Check sheet for the modelled part. Datum: model origin and axes. Units: mm. Face numbers are marked on the shaded views. A direction names the side the tool comes from. Round coordinates to 2 decimals unless told otherwise and drop trailing zeros. Order: outer loops, then holes, each group sorted by start corner. A loop starts at its lowest first (then second) coordinate and runs counter-clockwise, first axis right, second up. Notation, with made-up numbers: M -25,-18.75 L -17,-18.75 A12 ccw -17,-3.75 Z; hole C 61.5,79.25 d3. An arc over 180 degrees is marked long. One line per item, written item: value. Start each with the question number.
(1) Thickness scan on L1, parallel to X at y = 0, z = 14.5; L2, parallel to X at y = 3, z = 11; L3, parallel to X at y = -0.75, z = 30. Record the ranges inside material, lowest first.
(2) Depth check by flat-ended pin: pin 1 Ø7 at (x, y) = (20, 0) entering from -Z; pin 2 Ø3 at (x, y) = (-1.5, -0.5) entering from -Z. Enter the tip coordinate at first touch or a pass-through.
(3) Cross-section at B-B, the plane y = 0. Enter the section's corners in (x, z), and give its area (3 significant figures).
(4) Cross-section at D-D, the plane y = 4. Enter the section's corners in (x, z).
(5) Cross-section at A-A, the plane z = 14.5. Enter the section's corners in (x, y).
(6) Release check for a two-part mould opening along Y. For the marked faces 3, 4 and 5 record: released by +Y, released by -Y, zero draft, split by the parting line, or undercut.
(7) Access from +Z, -Z, +X, -X, +Y, -Y to the whole of each face (thin tool, end or side, straight path). Record for the marked faces 1 and 2.
(8) Cross-section at C-C, the plane x = 21. Enter the section's corners in (y, z).
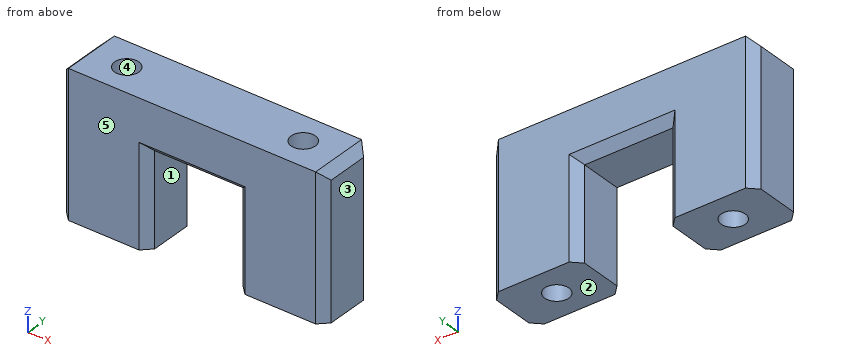
from build123d import *

# Parameters (mm, degrees)
SKETCH1_W           = 13.5
SKETCH1_H           = 60
SKETCH1_R           = 2.75
BOSS_EXTRUDE1_DEPTH = 32.5
SKETCH2_W           = 20
SKETCH2_H           = 21
CUT_EXTRUDE1_DEPTH  = 14.5
CHAMFER1_SIZE       = 2
CHAMFER2_SIZE       = 2


with BuildPart() as part:
    # Sketch1 → Boss-Extrude1 (new body)
    with BuildSketch(Plane(origin=(0, 0, 0), x_dir=(0, 1, 0), z_dir=(0, 0, 1))):
        Rectangle(SKETCH1_W, SKETCH1_H)
        with Locations((0, 20)):
            Circle(SKETCH1_R, mode=Mode.SUBTRACT)
        with Locations((0, -20)):
            Circle(SKETCH1_R, mode=Mode.SUBTRACT)
    extrude(amount=BOSS_EXTRUDE1_DEPTH)

    # Sketch2 → Cut-Extrude1 (cut, through all)
    with BuildSketch(Plane(origin=(0, 6.75, 0), x_dir=(-1, 0, 0), z_dir=(0, 1, 0))):
        with Locations((0, 10.5)):
            Rectangle(SKETCH2_W, SKETCH2_H)
    extrude(amount=-CUT_EXTRUDE1_DEPTH, mode=Mode.SUBTRACT)

    # Chamfer1
    chamfer1_edges = [part.edges().sort_by_distance(p)[0] for p in [
        (30, 0, 32.5),
        (30, 6.75, 16.25),
        (30, -6.75, 16.25),
        (-30, -6.75, 16.25),
        (-30, 6.75, 16.25),
        (-30, 0, 32.5),
    ]]
    chamfer(chamfer1_edges, length=CHAMFER1_SIZE)

    # Chamfer2
    chamfer2_edges = [part.edges().sort_by_distance(p)[0] for p in [
        (10, -6.75, 10.5),
        (0, -6.75, 21),
        (-10, -6.75, 10.5),
        (10, 6.75, 10.5),
        (-10, 6.75, 10.5),
        (0, 6.75, 21),
    ]]
    chamfer(chamfer2_edges, length=CHAMFER2_SIZE)


solid = part.part
Values found:
1. L1: -30 to -22.75, -17.25 to -10, 10 to 17.25, 22.75 to 30
1. L2: -30 to -10, 10 to 30
1. L3: -30 to -22.65, -17.35 to 17.35, 22.65 to 30
2. pin 1: z = 0
2. pin 2: z = 21
3. outline: M -30,0 L -22.75,0 L -22.75,32.5 L -28,32.5 L -30,30.5 Z; M -17.25,0 L -10,0 L -10,21 L 10,21 L 10,0 L 17.25,0 L 17.25,32.5 L -17.25,32.5 Z; M 22.75,0 L 30,0 L 30,30.5 L 28,32.5 L 22.75,32.5 Z
3. area: 1,170 mm^2
4. outline: M -30,0 L -10,0 L -10,21 L 10,21 L 10,0 L 30,0 L 30,30.5 L 28,32.5 L -28,32.5 L -30,30.5 Z
5. outline: M -30,-4.75 L -28,-6.75 L -12,-6.75 L -10,-4.75 L -10,4.75 L -12,6.75 L -28,6.75 L -30,4.75 Z; M 10,-4.75 L 12,-6.75 L 28,-6.75 L 30,-4.75 L 30,4.75 L 28,6.75 L 12,6.75 L 10,4.75 Z; hole C -20,0 d5.5; hole C 20,0 d5.5
6. face 3: zero draft
6. face 4: undercut
6. face 5: released by -Y
7. face 1: -Z, +Y, -Y
7. face 2: -Z, +X, -X, +Y, -Y
8. outline: M -6.75,0 L -2.56,0 L -2.56,32.5 L -6.75,32.5 Z; M 2.56,0 L 6.75,0 L 6.75,32.5 L 2.56,32.5 Z
